Read the model definition and answer for the solid it produces. Units are mm, in the model's axes. Face numbers are marked on the shaded views. A direction names the side the tool comes from. Coordinates: 2 decimals unless noted, no trailing zeros. Write each loop counter-clockwise with the first axis right and the second up, starting at its lowest first coordinate (ties: lowest second). Pieces come first, ordered by that corner, then holes.
(1) Section B-B on x = 0 is taken. Write down the section's boundary in (y, z), then the cut area to 4 significant figures.
(2) Section C-C on y = -1.75 is taken. State how many separate pieces and enclosed holes the cut face has, then the cut area to 3 significant figures.
(3) Find the intervals of material crossed by probe 1 along X at (y, z) = (-4.25, 0); probe 2 along Y at (x, z) = (-6.5, 18.5); probe 3 along X at (y, z) = (-2, -4), in increasing order.
(4) Given pin 1 (2.5 mm diameter, centred on x = -15.76, z = 10.61, fed in from +Y); pin 2 (6.5 mm diameter, centred on x = -1.5, z = -5, fed in from -Y); pin 3 (2 mm diameter, centred on y = -7, z = 12, fed in from +X); pin 4 (5 mm diameter, centred on x = 7, y = -3, fed in from +Z), each flat-ended and moving along its own axis, determine where each tip first touches the part or whether it passes through.
(5) The mould has two halves that part along Z. Classify the marked faces 1, 2, 3 and 4: +Z half, -Z half, draft (parallel to the pull), parting line (faces both ways), or undercut.
(6) Section D-D on x = 7.5 is taken. Write down the section's boundary in (y, z), then the cut area to 3 significant figures.
(7) Section A-A on z = 0 is taken. Write down the section's boundary in (x, y), then the cut area to 4 significant figures.
(8) Which of the six approach directions +Z, -Z, +X, -X, +Y, -Y give full straight-line access (tool end or side, diameter ignored) to the marked faces 5 and 6?
from build123d import *

# Parameters (mm, degrees)
DIAM_TRE_DU_PER_AGE_3_0_3_1_D = 3


with BuildPart() as part:
    # Esquisse1 → R_volution1 (revolve)
    with BuildSketch(Plane.XY, mode=Mode.PRIVATE) as r_volution1_sk:
        Polygon((-5.5, 0), (-22, 0), (-22, -5), (-15, -5), (-15, -11), (-11, -11), (-11, -8.5), (-5.5, -8.5), align=None)
    revolve(r_volution1_sk.sketch.rotate(Axis((0, 41.470120614, 0), (0, -1, 0)), 270), axis=Axis((0, 41.470120614, 0), (0, -1, 0)))

    # Diam_tre du per_age _3.0 _3_1 (through all)
    with Locations(Plane(origin=(3.647024388, 0, -18.646694429), x_dir=(0, 0, 1), z_dir=(0, 1, 0))):
        with Locations((0, 0), (8.05893299, 12.12951857), (22.320944817, 14.994324385), (2.934102993, -14.329461861), (14.999670041, -22.293718817), (29.25306283, -19.411064141), (37.293388858, -7.294048776), (34.410734182, 6.959344013)):
            Hole(DIAM_TRE_DU_PER_AGE_3_0_3_1_D / 2)


solid = part.part
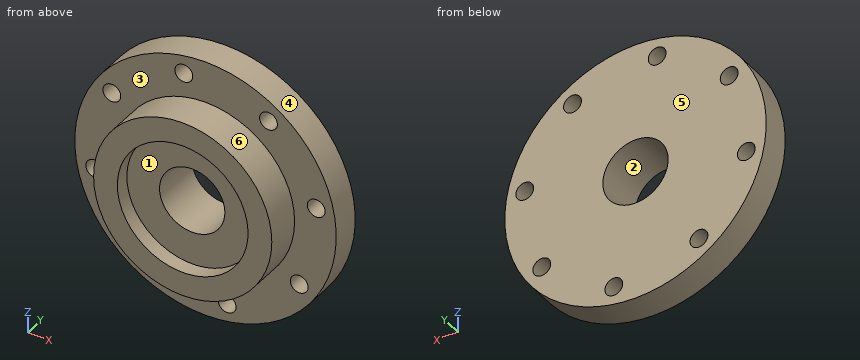
Response:
1. outline: (-11, -15) - (-5, -15) - (-5, -22) - (0, -22) - (0, -5.5) - (-8.5, -5.5) - (-8.5, -11) - (-11, -11) - close; (-11, 11) - (-8.5, 11) - (-8.5, 5.5) - (0, 5.5) - (0, 22) - (-5, 22) - (-5, 15) - (-11, 15) - close
1. area: 251.5 mm2
2. separate pieces: 1
2. enclosed holes: 9
2. area: 1,370 mm2
3. probe 1: x = -22 to -5.5, 5.5 to 22
3. probe 2: y = -5 to 0
3. probe 3: x = -21.63 to -20.1, -17.19 to -3.77, 3.77 to 21.63
4. pin 1: passes through
4. pin 2: stops at y = -8.5
4. pin 3: stops at x = 10.2
4. pin 4: stops at z = 21.53
5. face 1: undercut
5. face 2: undercut
5. face 3: draft
5. face 4: parting line
6. outline: (-11, -12.99) - (-5, -12.99) - (-5, -20.68) - (0, -20.68) - (0, 20.68) - (-5, 20.68) - (-5, 12.99) - (-11, 12.99) - (-11, 8.05) - (-8.5, 8.05) - (-8.5, -8.05) - (-11, -8.05) - close
6. area: 322 mm2
7. outline: (-22, -5) - (-15, -5) - (-15, -11) - (-11, -11) - (-11, -8.5) - (-5.5, -8.5) - (-5.5, 0) - (-22, 0) - close; (5.5, -8.5) - (11, -8.5) - (11, -11) - (15, -11) - (15, -5) - (22, -5) - (22, 0) - (5.5, 0) - close
7. area: 251.5 mm2
8. face 5: +Z, -Z, +X, -X, +Y
8. face 6: -Y
